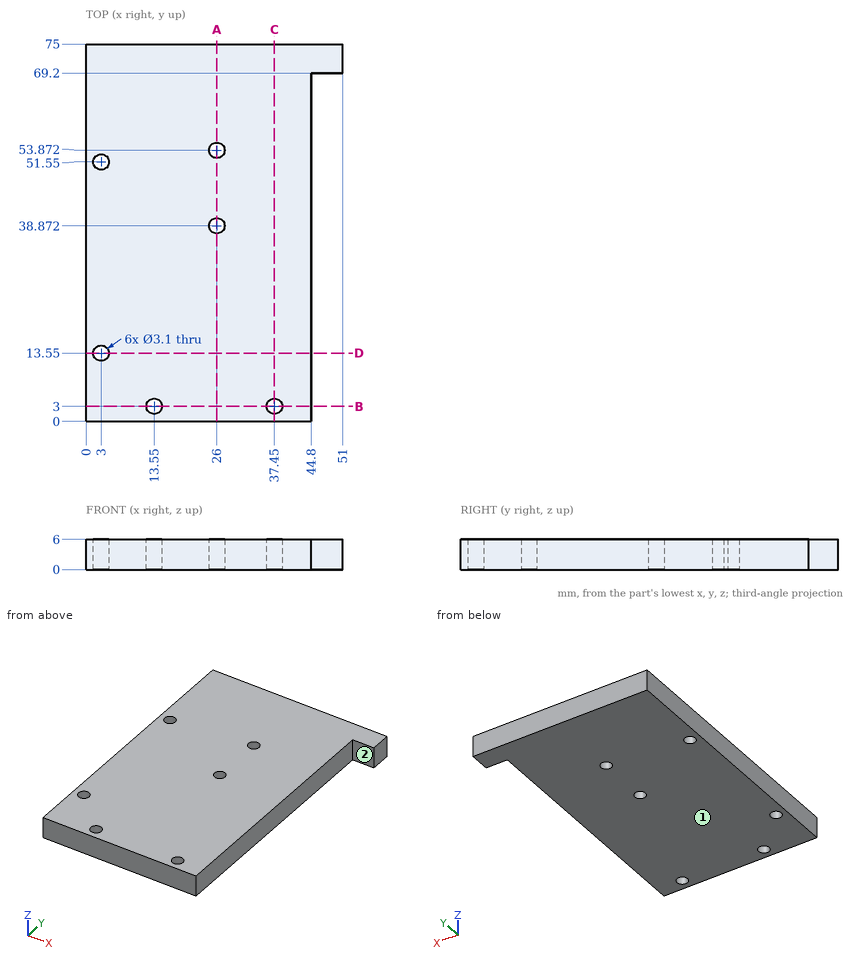
Verification items for this drawing (mm, ordinates from the low corner). A direction names the side the tool comes from. Round coordinates to 2 decimals unless told otherwise and drop trailing zeros. Loops run counter-clockwise (first coordinate to the right, second up) from the corner with the lowest first, then second, coordinate; pieces in that order, holes last. Notation, with made-up numbers: (-2, 21.25) -> (8, 21.25) arc R9 cw to (8, 30.25) -> close; hole circle Ø11 at (33.5, 23.5). An arc over 180 degrees is marked (long way). Write item = value, one per line. Start each with the question number.
1) Sectioned sample at A-A, the plane x = 26. Record the cut outline in (y, z), plus the area to 3 significant figures.
2) Thickness scan on probe 1 along Y at (x, z) = (3, 3.1); probe 2 along Y at (x, z) = (26, 3.9); probe 3 along Y at (x, z) = (37.45, 3.8). Record the ranges inside material, lowest first.
3) Sectioned sample at C-C, the plane x = 37.45. Record the cut outline in (y, z), plus the area to 3 significant figures.
4) Sectioned sample at D-D, the plane y = 13.55. Record the cut outline in (x, z), plus the area to 3 significant figures.
5) Sectioned sample at B-B, the plane y = 3. Record the cut outline in (x, z), plus the area to 3 significant figures.
6) Gauge pin test, flat end, axial feed: pin 1 Ø1.8 at (y, z) = (26.5, 4.5) entering from +X. Record the tip position at first contact, or that the pin passes through.
7) Set-up check for the marked faces 1 and 2: record each of +Z, -Z, +X, -X, +Y, -Y from which the full face is reachable in a straight line by a thin tool's end or side.
Results are:
q1.outline = (0, 0) -> (37.32, 0) -> (37.32, 6) -> (0, 6) -> close; (40.42, 0) -> (52.32, 0) -> (52.32, 6) -> (40.42, 6) -> close; (55.42, 0) -> (75, 0) -> (75, 6) -> (55.42, 6) -> close
q1.area = 413 mm^2
q2.probe_1 = 0 to 12, 15.1 to 50, 53.1 to 75
q2.probe_2 = 0 to 37.32, 40.42 to 52.32, 55.42 to 75
q2.probe_3 = 0 to 1.45, 4.55 to 75
q3.outline = (0, 0) -> (1.45, 0) -> (1.45, 6) -> (0, 6) -> close; (4.55, 0) -> (75, 0) -> (75, 6) -> (4.55, 6) -> close
q3.area = 431 mm^2
q4.outline = (0, 0) -> (1.45, 0) -> (1.45, 6) -> (0, 6) -> close; (4.55, 0) -> (44.8, 0) -> (44.8, 6) -> (4.55, 6) -> close
q4.area = 250 mm^2
q5.outline = (0, 0) -> (12, 0) -> (12, 6) -> (0, 6) -> close; (15.1, 0) -> (35.9, 0) -> (35.9, 6) -> (15.1, 6) -> close; (39, 0) -> (44.8, 0) -> (44.8, 6) -> (39, 6) -> close
q5.area = 232 mm^2
q6.pin_1 = 44.8
q7.face_1 = -Z, +X, -X, +Y, -Y
q7.face_2 = +Z, -Z, +X, -Y
